Autodesk Inventor part; units mm, degrees
ref_plane "YZ Plane" through (0, 0, 0) normal (1, 0, 0) x (0, 1, 0)
ref_plane "XZ Plane" through (0, 0, 0) normal (0, 1, 0) x (-1, 0, 0)
ref_plane "XY Plane" through (0, 0, 0) normal (0, 0, 1) x (1, 0, 0)
ref_plane "Work Plane1" through (24.9, 0, 1) normal (0, 0, 1) x (1, 0, 0)
sketch "Sketch1" plane through (24.9, 0, 1) normal (0, 0, 1) x (1, 0, 0)
  circle A0 centre (-55.5143, -4) radius 2.45
  circle A1 centre (-30.5143, -4) radius 2.45
  circle A2 centre (-30.5143, -20) radius 2.45
  line L0 (-55.5143, -4) -> (-30.5143, -4)
  line L1 (-30.5143, -4) -> (-30.5143, -20)
  line L2 (-30.5143, -20) -> (-55.5143, -20)
  line L3 (-55.5143, -20) -> (-55.5143, -4)
  line L4 (-27.5143, -1) -> (-58.5143, -1)
  line L5 (-58.5143, -1) -> (-58.5143, -23)
  line L6 (-58.5143, -23) -> (-27.5143, -23)
  line L7 (-27.5143, -23) -> (-27.5143, -1)
  circle A3 centre (-55.5143, -4) radius 1.4
  circle A4 centre (-30.5143, -4) radius 1.4
  circle A5 centre (-30.5143, -20) radius 1.4
  circle A6 centre (-55.5143, -20) radius 1.4
  dimension "d0" = 4.9
  dimension "d1" = 4.9
  dimension "d2" = 4.9
  dimension "d3" = 3
extrude "Extrusion1" add sketch "Sketch1" along normal blind 3.5 contours L0 A1 L1 A2 L2 A6 L3 A0 | L7 L6 L5 L4
sketch "Sketch2" plane through (24.9, 0, 4.5) normal (0, 0, 1) x (1, 0, 0)
  circle A0 centre (-30.5143, -4) radius 2.45
  circle A1 centre (-30.5143, -20) radius 2.45
  circle A2 centre (-55.5143, -4) radius 2.45
  line L0 (-58.5143, -1) -> (-58.5143, -23)
  line L1 (-58.5143, -23) -> (-27.5143, -23)
  line L2 (-27.5143, -23) -> (-27.5143, -1)
  line L3 (-27.5143, -1) -> (-58.5143, -1)
  circle A3 centre (-55.5143, -20) radius 1.4
  circle A4 centre (-30.5143, -20) radius 2.45
  circle A5 centre (-30.5143, -4) radius 2.45
  circle A6 centre (-55.5143, -4) radius 2.45
  point P0 (-24.9, 0)
extrude "Extrusion2" add sketch "Sketch2" along normal blind 1 contours A0 | A1 | A2 | L3 L2 L1 L0 | A3
fillet "Fillet1" radius 2 4 edges at (-33.6143, -23, 3.25) (-2.6143, -23, 3.25) (-33.6143, -1, 3.25) (-2.6143, -1, 3.25)
equation "\"d1\" = d0"
equation "\"d2\" = d0"
properties part number "20_Cube_4_insert_Lens_kinematic_mirrormount_plate"
Input: part model. Units: mm. Frame: model coordinates. A direction names the side the tool comes from. Round coordinates to 2 decimals unless told otherwise and drop trailing zeros. Write each loop counter-clockwise with the first axis right and the second up, starting at its lowest first coordinate (ties: lowest second). Pieces come first, ordered by that corner, then holes.
1) Reachability of faces 1 (the flat face through (-18, -12, 5.5)), 2 (the flat face through (-6, -4, 4.5)) from +Z, -Z, +X, -X, +Y, -Y: full face, straight path, thin tool, end or side. Return the list, or none.
2) Cut plane B-B (y = -4). Return the cut outline in (x, z), then the cut area to 3 significant figures.
3) Cut plane A-A (z = 1.8). Return the cut outline in (x, y), then the cut area to 3 significant figures.
4) Ray query, L1, parallel to X at y = -4, z = 2.2; L2, parallel to X at y = -20, z = 3.7; L3, parallel to X at y = -18.5, z = 3.45. Return the intervals inside material, ascending.
5) Cut plane C-C (y = -20). Return the cut outline in (x, z), then the cut area to 3 significant figures.
6) Contact query for a flat-ended pin moving along its axis: P1, Ø4, axis at x = -30.61, y = -4, coming from the -Z side. Output: stop coordinate, or through.
7) Draft query along X for faces 3 (the cylindrical face through (-33.04, -22.4, 3.28)), 4 (the flat face through (-2.614, -12, 3)), 5 (the flat face through (-31, -4, 4.5)). Return one class per face: pulls with the +X half, pulls with the -X half, needs draft (parallel to the pull), parting line crosses it, or undercut.
Geometry says:
1. face 1: +Z, +X, -X, +Y, -Y
1. face 2: -Z
2. outline: (-33.61, 1) - (-33.06, 1) - (-33.06, 4.5) - (-28.16, 4.5) - (-28.16, 1) - (-8.06, 1) - (-8.06, 4.5) - (-3.16, 4.5) - (-3.16, 1) - (-2.61, 1) - (-2.61, 5.5) - (-33.61, 5.5) - close
2. area: 105 mm2
3. outline: (-33.61, -21) arc R2 ccw to (-31.61, -23) - (-4.61, -23) arc R2 ccw to (-2.61, -21) - (-2.61, -3) arc R2 ccw to (-4.61, -1) - (-31.61, -1) arc R2 ccw to (-33.61, -3) - close; hole circle Ø4.9 at (-30.61, -4); hole circle Ø2.8 at (-30.61, -20); hole circle Ø4.9 at (-5.61, -20); hole circle Ø4.9 at (-5.61, -4)
3. area: 616 mm2
4. L1: x = -33.61 to -33.06, -28.16 to -8.06, -3.16 to -2.61
4. L2: x = -33.61 to -32.01, -29.21 to -8.06, -3.16 to -2.61
4. L3: x = -33.61 to -7.55, -3.68 to -2.61
5. outline: (-33.61, 1) - (-32.01, 1) - (-32.01, 4.5) - (-29.21, 4.5) - (-29.21, 1) - (-8.06, 1) - (-8.06, 4.5) - (-3.16, 4.5) - (-3.16, 1) - (-2.61, 1) - (-2.61, 5.5) - (-33.61, 5.5) - close
5. area: 113 mm2
6. P1: stops at z = 4.5
7. face 3: pulls with the -X half
7. face 4: pulls with the +X half
7. face 5: undercut
